The listing builds one solid part. Answer for the finished solid, in the listing's coordinates (mm). Face numbers are marked on the shaded views. A direction names the side the tool comes from. Give positions to 0.01 mm unless a question says otherwise; leave off trailing zeros. Order: outer loops, then holes, each group sorted by start corner. A loop starts at its lowest first (then second) coordinate and runs counter-clockwise, first axis right, second up. Notation, with made-up numbers: M 44,40.25 L 98,40.25 A11 ccw 98,57.25 Z; hole C 38,60 d4. An arc over 180 degrees is marked long. Answer as a JSON object with one key per item and string values. Group by question number.
```python
from build123d import *

# Parameters (mm, degrees)
F1_DEPTH = 25.4


with BuildPart() as f1:
    # F0 (on Front) → F1 (new body)
    with BuildSketch(Plane.XZ):
        with BuildLine():
            ThreePointArc((-22.036027, -44.072051), (-9.67173, -47.480311), (0, -55.903476))
            Line((0, -55.903476), (35.050593, -25.733344))
            Line((35.050593, -25.733344), (27.95174, -25.733344))
            Line((27.95174, -25.733344), (57.84783, 0))
            Line((57.84783, 0), (51.614583, 0))
            Line((51.614583, 0), (57.84783, 5.365327))
            ThreePointArc((57.84783, 5.365327), (35.136908, 10.627208), (11.979315, 13.310351))
            ThreePointArc((11.979315, 13.310351), (-1.03525, 24.439791), (-14.049816, 13.310351))
            ThreePointArc((-14.049816, 13.310351), (-28.935956, 12.342824), (-43.628372, 9.760925))
            Line((-43.628372, 9.760925), (-41.26209, 6.211497))
            ThreePointArc((-41.26209, 6.211497), (-53.555536, 2.447613), (-65.220721, -2.957856))
            Line((-65.220721, -2.957856), (-56.05137, -15.972422))
            Line((-56.05137, -15.972422), (-38.008448, -26.620703))
            Line((-38.008448, -26.620703), (-33.895824, -24.204055))
            ThreePointArc((-33.895824, -24.204055), (-27.665097, -23.432097), (-22.833852, -27.441703))
            ThreePointArc((-22.833852, -27.441703), (-21.387026, -29.099123), (-19.326398, -29.869942))
            ThreePointArc((-19.326398, -29.869942), (-16.78065, -28.362967), (-16.628357, -25.408544))
            ThreePointArc((-16.628357, -25.408544), (-9.613447, -24.476899), (-2.598537, -25.408544))
            ThreePointArc((-2.598537, -25.408544), (-4.681451, -27.595484), (-7.455012, -28.790725))
            ThreePointArc((-7.455012, -28.790725), (-11.255149, -29.946665), (-13.66051, -33.107594))
            ThreePointArc((-13.66051, -33.107594), (-16.238261, -35.131125), (-13.66051, -37.154656))
            ThreePointArc((-13.66051, -37.154656), (-19.596203, -39.078416), (-25.531895, -37.154656))
            ThreePointArc((-25.531895, -37.154656), (-24.252791, -39.840887), (-21.484831, -40.931914))
            Line((-21.484831, -40.931914), (-25.531895, -40.931914))
            Line((-25.531895, -40.931914), (-22.036027, -44.072051))
        make_face()
        with BuildLine():
            ThreePointArc((-11.203147, 11.265573), (-1.03525, 21.43347), (9.132647, 11.265573))
            ThreePointArc((9.132647, 11.265573), (-1.03525, 12.94309), (-11.203147, 11.265573))
        make_face(mode=Mode.SUBTRACT)
    extrude(amount=F1_DEPTH)


solid = f1.part
```
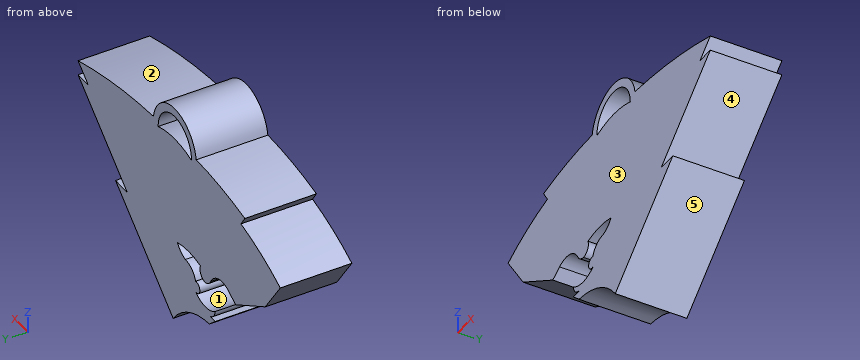
Item 1: Determine the mould class of the marked faces 1, 2 and 3 for opening direction X: released by +X, released by -X, zero draft, split by the parting line, or undercut.
Item 2: Section D-D (x = 19.5) is taken. Determine the outline of the cut face in (y, z), and give its area (3 significant figures).
Item 3: Flat-ended cylindrical pins translate along their axes: P1, Ø2, axis at x = 21, y = -21.5, coming from the -Z side; P2, Ø12, axis at y = -18, z = -11.5, coming from the -X side; P3, Ø10, axis at x = 30.5, y = -20, coming from the -Z side. Find the tip coordinate at first contact, or state that the pin passes through.
Item 4: Section B-B (x = 5) is taken. Determine the outline of the cut face in (y, z).
Item 5: Section C-C (z = -9) is taken. Determine the outline of the cut face in (x, y).
Item 6: Section A-A (y = -16.5) is taken. Determine the outline of the cut face in (x, z).
Item 7: A tool of negligible diameter and unlimited length cuts with its end or side. For the marked faces 4 and 5, from which of +Z, -Z, +X, -X, +Y, -Y can it reach the whole face along a straight path? Write none if from no direction.
Item 8: Consider probe 1 along X at (y, z) = (-15, 14.5) (1 decimal); probe 2 along Z at (x, y) = (-17, -22); probe 3 along Z at (x, y) = (-12, -2.75). Determine where each line is inside the solid, lowest interval first. Write a range as from..to.
Values found:
{
 "1": {"face 1": "undercut", "face 2": "released by +X", "face 3": "zero draft"},
 "2": {"outline": "M -25.4,-39.12 L 0,-39.12 L 0,12.73 L -25.4,12.73 Z", "area": "1,320 mm^2"},
 "3": {"P1": "stops at z = -38.69", "P2": "stops at x = -63.43", "P3": "stops at z = -33.95"},
 "4": {"outline": "M -25.4,-51.6 L 0,-51.6 L 0,12.36 L -25.4,12.36 Z; M -25.4,19.45 L 0,19.45 L 0,22.98 L -25.4,22.98 Z"},
 "5": {"outline": "M -60.96,-25.4 L 47.39,-25.4 L 47.39,0 L -60.96,0 Z"},
 "6": {"outline": "M -65.22,-2.96 L -56.05,-15.97 L -38.01,-26.62 L -33.9,-24.2 A7.91 cw -22.83,-27.44 A4.49 ccw -19.33,-29.87 A3.13 ccw -16.63,-25.41 A26.88 cw -2.6,-25.41 A7.55 cw -7.46,-28.79 A6.46 ccw -13.66,-33.11 A2.08 ccw long -13.66,-37.15 A10.12 cw -25.53,-37.15 A4.06 ccw -21.48,-40.93 L -25.53,-40.93 L -22.04,-44.07 A28.9 cw 0,-55.9 L 35.05,-25.73 L 27.95,-25.73 L 57.85,0 L 51.61,0 L 57.85,5.37 A207.66 ccw 11.98,13.31 A13.17 ccw -14.05,13.31 A136.86 ccw -43.63,9.76 L -41.26,6.21 A94.04 ccw Z; hole M -11.2,11.27 A31.65 cw 9.13,11.27 A10.17 ccw Z"},
 "7": {"face 4": "+X, +Y, -Y", "face 5": "-Z, +X, +Y, -Y"},
 "8": {"probe 1": "x = -13.8..-10.7, 8.6..11.7", "probe 2": "z = -44.75..-38.74, -28.68..13.25", "probe 3": "z = -46.36..-30.55, -24.58..18.57"}
}
